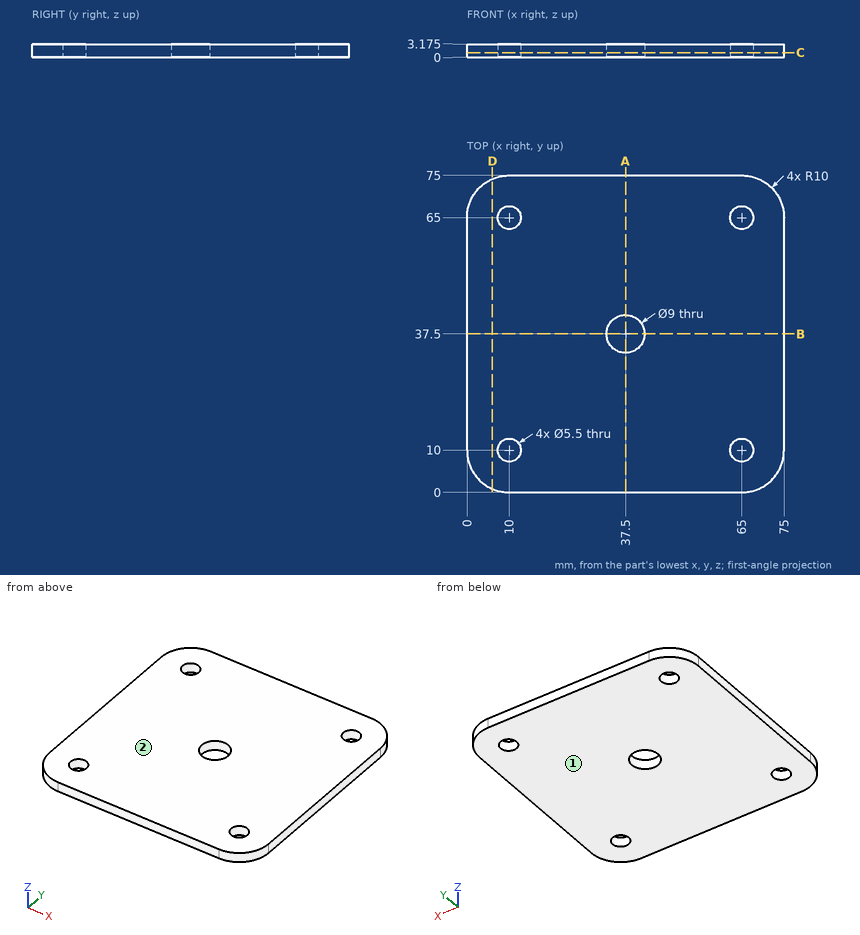
Source: three-view drawing plus pictorial views. Frame: mm from the lowest corner of the part. Give positions to 0.01 mm unless a question says otherwise; leave off trailing zeros. Order: outer loops, then holes, each group sorted by start corner. A loop starts at its lowest first (then second) coordinate and runs counter-clockwise, first axis right, second up. Notation, with made-up numbers: M -13.75,-36 L 4.25,-36 A14 ccw 4.25,-28 Z; hole C 68,26 d2. An arc over 180 degrees is marked long. Return JSON: item names as keys, results as strings.
1) Section query A-A on x = 37.5. Output: boundary loops of the cut face in (y, z) (3 decimals).
Taken from the geometry:
{"outline": "M 0,0 L 33,0 L 33,3.175 L 0,3.175 Z; M 42,0 L 75,0 L 75,3.175 L 42,3.175 Z"}
2) Section query C-C on z = 1.15. Output: boundary loops of the cut face in (x, y).
Taken from the geometry:
{"outline": "M 0,10 A10 ccw 10,0 L 65,0 A10 ccw 75,10 L 75,65 A10 ccw 65,75 L 10,75 A10 ccw 0,65 Z; hole C 10,10 d5.5; hole C 10,65 d5.5; hole C 37.5,37.5 d9; hole C 65,10 d5.5; hole C 65,65 d5.5"}
3) Line query: L1, parallel to Y at x = 10, z = 2.55; L2, parallel to X at y = 38, z = 0.8; L3, parallel to Y at x = 66, z = 2.05. Output: solid intervals per line, ascending. Write a range as [from, to].
Taken from the geometry:
{"L1": "y = [0, 7.25], [12.75, 62.25], [67.75, 75]", "L2": "x = [0, 33.03], [41.97, 75]", "L3": "y = [0.05, 7.44], [12.56, 62.44], [67.56, 74.95]"}
4) Section query D-D on x = 6. Output: boundary loops of the cut face in (y, z) (3 decimals).
Taken from the geometry:
{"outline": "M 0.835,0 L 74.165,0 L 74.165,3.175 L 0.835,3.175 Z"}
5) Mould query, pull axis Z, two halves, no side actions, for the marked faces 1 and 2. Classes: released by +Z, released by -Z, zero draft, split by the parting line, or undercut.
Taken from the geometry:
{"face 1": "released by -Z", "face 2": "released by +Z"}
6) Contact query for a flat-ended pin moving along its axis: pin 1 (5.5 mm diameter, centred on x = 37.5, y = 37.5, fed in from -Z). Output: stop coordinate, or through.
Taken from the geometry:
{"pin 1": "passes through"}
